Geometry check sheet. Reference: the model listing, model coordinates, mm. Give positions to 0.01 mm unless a question says otherwise; leave off trailing zeros. Loops run counter-clockwise (first coordinate to the right, second up) from the corner with the lowest first, then second, coordinate; pieces in that order, holes last. Notation, with made-up numbers: (-12.5, -16) - (21.5, -16) arc R17 cw to (21.5, 2) - close; hole circle Ø1 at (16.5, -36.5). An arc over 180 degrees is marked (long way). One line per question, with ' | ' between items. Start each with the question number.
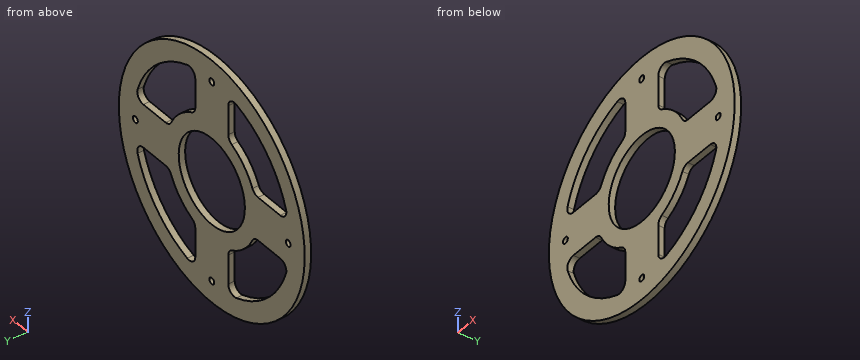
from build123d import *

# Parameters (mm, degrees)
BOSS_EXTRUDE1_DEPTH      = 2
BOSS_EXTRUDE1_DEPTH_BACK = 2
SKETCH1_R                = 76
SKETCH1_R_2              = 27.051
SKETCH1_R_3              = 2
CUT_EXTRUDE2_DEPTH       = 108.554637278
FILLET1_R                = 5


with BuildPart() as part:
    # Sketch1 → Boss-Extrude1 (new, two sides: drawn at the far end of the back side and taken through both)
    with BuildSketch(Plane(origin=(0, 0, 0), x_dir=(1, 0, 0), z_dir=(0, 1, 0)).offset(-BOSS_EXTRUDE1_DEPTH_BACK)):
        with Locations(Location((0, 0, 0), (0, 0, 270))):
            Circle(SKETCH1_R)
        with Locations(Location((0, 0, 0), (0, 0, 270))):
            Circle(SKETCH1_R_2, mode=Mode.SUBTRACT)
        with Locations(Location((0, 62.5, 0), (0, 0, 270))):
            Circle(SKETCH1_R_3, mode=Mode.SUBTRACT)
        with Locations(Location((62.5, 0, 0), (0, 0, 270))):
            Circle(SKETCH1_R_3, mode=Mode.SUBTRACT)
        with Locations(Location((0, -62.5, 0), (0, 0, 270))):
            Circle(SKETCH1_R_3, mode=Mode.SUBTRACT)
        with Locations(Location((-62.5, 0, 0), (0, 0, 270))):
            Circle(SKETCH1_R_3, mode=Mode.SUBTRACT)
    extrude(amount=BOSS_EXTRUDE1_DEPTH + BOSS_EXTRUDE1_DEPTH_BACK)

    # Sketch4 → Cut-Extrude2 (cut, through all)
    with BuildSketch(Plane(origin=(0, 2, 0), x_dir=(1, 0, 0), z_dir=(0, 1, 0))):
        with BuildLine():
            ThreePointArc((-34.504008477, 13.5), (-26.19901335, 26.19901335), (-13.5, 34.504008477))
            Line((-13.5, 34.504008477), (-13.5, 62.5))
            ThreePointArc((-13.5, 62.5), (-45.213382975, 45.213382975), (-62.5, 13.5))
            Line((-62.5, 13.5), (-34.504008477, 13.5))
        make_face()
        with BuildLine():
            ThreePointArc((62.5, 13.5), (45.213382975, 45.213382975), (13.5, 62.5))
            Line((13.5, 62.5), (13.5, 34.504008477))
            ThreePointArc((13.5, 34.504008477), (26.19901335, 26.19901335), (34.504008477, 13.5))
            Line((34.504008477, 13.5), (62.5, 13.5))
        make_face()
        with BuildLine():
            Line((62.5, -13.5), (34.504008477, -13.5))
            ThreePointArc((34.504008477, -13.5), (26.19901335, -26.19901335), (13.5, -34.504008477))
            Line((13.5, -34.504008477), (13.5, -62.5))
            ThreePointArc((13.5, -62.5), (45.213382975, -45.213382975), (62.5, -13.5))
        make_face()
        with BuildLine():
            ThreePointArc((-13.5, -34.504008477), (-26.19901335, -26.19901335), (-34.504008477, -13.5))
            Line((-34.504008477, -13.5), (-62.5, -13.5))
            ThreePointArc((-62.5, -13.5), (-45.213382975, -45.213382975), (-13.5, -62.5))
            Line((-13.5, -62.5), (-13.5, -34.504008477))
        make_face()
    extrude(amount=-CUT_EXTRUDE2_DEPTH, mode=Mode.SUBTRACT)

    # Fillet1
    fillet1_edges = [part.edges().sort_by_distance(p)[0] for p in [
        (-34.504008477, 0, 13.5),
        (-13.5, 0, 34.504008477),
        (-13.5, 0, 62.5),
        (-62.5, 0, 13.5),
        (13.5, 0, 34.504008477),
        (34.504008477, 0, 13.5),
        (62.5, 0, 13.5),
        (13.5, 0, 62.5),
        (34.504008477, 0, -13.5),
        (13.5, 0, -34.504008477),
        (13.5, 0, -62.5),
        (62.5, 0, -13.5),
        (-13.5, 0, -34.504008477),
        (-34.504008477, 0, -13.5),
        (-62.5, 0, -13.5),
        (-13.5, 0, -62.5),
    ]]
    fillet(fillet1_edges, radius=FILLET1_R)


solid = part.part
(1) Section check A-A, the plane z = 0. Record the boundary of the cut face in (x, y).
(2) Depth check by flat-ended pin: pin 1 Ø1.2 at (y, z) = (1, 43) entering from +X; pin 2 Ø2 at (x, z) = (-23.5, -29) entering from +Y; pin 3 Ø1.5 at (y, z) = (-1.5, -27) entering from +X; pin 4 Ø1.2 at (x, y) = (-49, -1) entering from +Z. Enter the tip coordinate at first touch or a pass-through.
(3) Section check B-B, the plane x = -9. Record the boundary of the cut face in (y, z), and give its area (3 significant figures).
(4) Section check C-C, the plane x = 31. Record the boundary of the cut face in (y, z), and give its area (3 significant figures).
(5) Section check D-D, the plane y = 1.4. Count the separate pieces of the cut face and the enclosed holes in it, and give its area (3 significant figures).
(6) Material ranges on line 1 (X direction, y = 0.4, z = 0); line 2 (Z direction, x = -54, y = 1.7); line 3 (Z direction, x = 31.5, y = 1.25), recorded low to high.
Numbers:
1) outline: (-76, -2) - (-64.5, -2) - (-64.5, 2) - (-76, 2) - close; (-60.5, -2) - (-27.05, -2) - (-27.05, 2) - (-60.5, 2) - close; (27.05, -2) - (60.5, -2) - (60.5, 2) - (27.05, 2) - close; (64.5, -2) - (76, -2) - (76, 2) - (64.5, 2) - close
2) pin 1: x = 63.07 | pin 2: y = 2 | pin 3: x = 71.32 | pin 4: z = 58.6
3) outline: (-2, -75.47) - (2, -75.47) - (2, -25.51) - (-2, -25.51) - close; (-2, 25.51) - (2, 25.51) - (2, 75.47) - (-2, 75.47) - close | area: 400 mm^2
4) outline: (-2, -69.39) - (2, -69.39) - (2, -55.92) - (-2, -55.92) - close; (-2, -20.29) - (2, -20.29) - (2, 20.29) - (-2, 20.29) - close; (-2, 55.92) - (2, 55.92) - (2, 69.39) - (-2, 69.39) - close | area: 270 mm^2
5) separate pieces: 1 | enclosed holes: 9 | area: 10,300 mm^2
6) line 1: -76 to -64.5, -60.5 to -27.05, 27.05 to 60.5, 64.5 to 76 | line 2: -53.48 to -34.24, -13.5 to 13.5, 34.24 to 53.48 | line 3: -69.16 to -55.64, -19.51 to 19.51, 55.64 to 69.16
